```python
from build123d import *

# Parameters (mm, degrees)
EXTRUDE_3_DEPTH      = 5
EXTRUDE_4_DEPTH      = 25
EXTRUDE_4_DEPTH_BACK = 8
SKETCH_4_W           = 65
SKETCH_4_H           = 4
CUT_EXTRUDE_START    = -65
SKETCH_5_W           = 1.4
SKETCH_5_H           = 1.7
CUT_EXTRUDE_1_DEPTH  = 65
SKETCH_6_R           = 2
CUT_EXTRUDE_2_DEPTH  = 5
SKETCH_7_R           = 1.65
CUT_EXTRUDE_3_DEPTH  = 4


with BuildPart() as part:
    # 草图2 → 凸台-拉伸3 (new body)
    with BuildSketch(Plane(origin=(0, 0, 0), x_dir=(0, 0, -1), z_dir=(1, 0, 0))):
        Polygon((32.5, -19.5), (20.75, -19.5), (20.75, 4.5), (-20.75, 4.5), (-20.75, -19.5), (-32.5, -19.5), (-32.5, 19.5), (32.5, 19.5), align=None)
    extrude(amount=EXTRUDE_3_DEPTH)

    # 草图4 → 凸台-拉伸4 (add, two sides: drawn at the far end of the back side and taken through both)
    with BuildSketch(Plane.ZY.offset(-EXTRUDE_4_DEPTH_BACK)):
        with Locations((0, 17.5)):
            Rectangle(SKETCH_4_W, SKETCH_4_H)
    extrude(amount=EXTRUDE_4_DEPTH + EXTRUDE_4_DEPTH_BACK)

    # 草图5 → 切除-拉伸1 (cut)
    with BuildSketch(Plane.XY.offset(32.5).offset(CUT_EXTRUDE_START)):
        with Locations((0.7, -8.75)):
            Rectangle(SKETCH_5_W, SKETCH_5_H)
    extrude(amount=CUT_EXTRUDE_1_DEPTH, mode=Mode.SUBTRACT)

    # 草图6 → 切除-拉伸2 (cut)
    with BuildSketch(Plane(origin=(5, 0, 0), x_dir=(0, 0, -1), z_dir=(1, 0, 0))):
        with Locations((-25, -3.75)):
            Circle(SKETCH_6_R)
        with Locations((-25, -13.75)):
            Circle(SKETCH_6_R)
        with Locations(Location((25, -13.75, 0), (0, 0, 180))):
            Circle(SKETCH_6_R)
        with Locations(Location((25, -3.75, 0), (0, 0, 180))):
            Circle(SKETCH_6_R)
    extrude(amount=-CUT_EXTRUDE_2_DEPTH, mode=Mode.SUBTRACT)

    # 草图7 → 切除-拉伸3 (cut)
    with BuildSketch(Plane(origin=(0, 19.5, 0), x_dir=(1, 0, 0), z_dir=(0, 1, 0))):
        with Locations(Location((-19.35, -18.85, 0), (0, 0, 270))):
            Circle(SKETCH_7_R)
        with Locations(Location((-5.65, -18.85, 0), (0, 0, 270))):
            Circle(SKETCH_7_R)
        with Locations(Location((-19.35, 18.85, 0), (0, 0, 270))):
            Circle(SKETCH_7_R)
        with Locations(Location((-5.65, 18.85, 0), (0, 0, 270))):
            Circle(SKETCH_7_R)
    extrude(amount=-CUT_EXTRUDE_3_DEPTH, mode=Mode.SUBTRACT)


solid = part.part
```
For this review, take the finished solid that the model builds, in its own axes (mm). A direction names the side the tool comes from. Round coordinates to 2 decimals unless told otherwise and drop trailing zeros. Write each loop counter-clockwise with the first axis right and the second up, starting at its lowest first coordinate (ties: lowest second). Pieces come first, ordered by that corner, then holes. Notation, with made-up numbers: (50, 21) - (76, 21) arc R25 cw to (76, 33) - close; hole circle Ø11 at (-32, 6.5). An arc over 180 degrees is marked (long way). Answer as a JSON object with one key per item and string values.
1. We need section A-A on z = 18.85. Give the boundary of the cut face in (x, y), then the cut area to 3 significant figures.
Response values:
{"outline": "(-25, 15.5) - (-21, 15.5) - (-21, 19.5) - (-25, 19.5) - close; (-17.7, 15.5) - (-7.3, 15.5) - (-7.3, 19.5) - (-17.7, 19.5) - close; (-4, 15.5) - (0, 15.5) - (0, 4.5) - (5, 4.5) - (5, 15.5) - (8, 15.5) - (8, 19.5) - (-4, 19.5) - close", "area": "161 mm2"}
2. We need section C-C on x = -5.65. Give the boundary of the cut face in (y, z), then the cut area to 3 significant figures.
Response values:
{"outline": "(15.5, -32.5) - (19.5, -32.5) - (19.5, -20.5) - (15.5, -20.5) - close; (15.5, -17.2) - (19.5, -17.2) - (19.5, 17.2) - (15.5, 17.2) - close; (15.5, 20.5) - (19.5, 20.5) - (19.5, 32.5) - (15.5, 32.5) - close", "area": "234 mm2"}
3. We need section D-D on z = -11.5. Give the boundary of the cut face in (x, y).
Response values:
{"outline": "(-25, 15.5) - (0, 15.5) - (0, 4.5) - (5, 4.5) - (5, 15.5) - (8, 15.5) - (8, 19.5) - (-25, 19.5) - close"}
4. We need section B-B on x = 3. Give the boundary of the cut face in (y, z), then the cut area to 3 significant figures.
Response values:
{"outline": "(-19.5, -32.5) - (19.5, -32.5) - (19.5, 32.5) - (-19.5, 32.5) - (-19.5, 20.75) - (4.5, 20.75) - (4.5, -20.75) - (-19.5, -20.75) - close; hole circle Ø4 at (-13.75, -25); hole circle Ø4 at (-13.75, 25); hole circle Ø4 at (-3.75, -25); hole circle Ø4 at (-3.75, 25)", "area": "1,490 mm2"}
5. Draft analysis for pull direction Z (two halves, no side actions). For faces 5 (the face through (5, 6, 0)), 6 (the face through (-20.35, 17.53, 17.54)), state which applies: +Z half, -Z half, draft (parallel to the pull), parting line (faces both ways), or undercut.
Response values:
{"face 5": "draft", "face 6": "undercut"}
6. For pin 1 Ø0.8 at (y, z) = (-9, -28) entering from -X; pin 2 Ø1.9 at (y, z) = (-8.5, 28) entering from -X; pin 3 Ø4 at (x, z) = (-19.35, 18.85) entering from -Y, all flat-tipped, find the tip position at first contact; note any pin that passes through.
Response values:
{"pin 1": "stops at x = 1.4", "pin 2": "stops at x = 0", "pin 3": "stops at y = 15.5"}
7. To check wall thickness, follow line 1 along X through (y, z) = (17.8, 18.85); line 2 along Y through (x, z) = (1, 25); line 3 along Y through (x, z) = (2.7, 25). State the ranges of each line that lie inside material, in increasing order.
Response values:
{"line 1": "x = -25 to -21, -17.7 to -7.3, -4 to 8", "line 2": "y = -19.5 to -15.75, -11.75 to -9.6, -7.9 to -5.75, -1.75 to 19.5", "line 3": "y = -19.5 to -15.75, -11.75 to -5.75, -1.75 to 19.5"}
8. Tool access review of faces 1 (the face through (1.4, -9, 27)), 2 (the face through (0, 7, 0)), 3 (the face through (7, 15.5, 0)), 4 (the face through (2, -7, 20.75)): name each direction out of +Z, -Z, +X, -X, +Y, -Y from which nothing blocks a thin tool from reaching the whole face with its end or side.
Response values:
{"face 1": "+Z, -Z, -X", "face 2": "+Z, -Z, -X, -Y", "face 3": "+Z, -Z, +X, -Y", "face 4": "+X, -X, -Y"}
